from build123d import *

# Parameters (mm, degrees)
SKETCH_1_R      = 8.490267481
EXTRUDE_1_DEPTH = 2
SKETCH_2_R      = 1.25
EXTRUDE_2_DEPTH = 2.5


with BuildPart() as part:
    # Эскиз1 → Бобышка-Вытянуть1 (new body)
    with BuildSketch(Plane(origin=(0, 0, 0), x_dir=(1, 0, 0), z_dir=(0, 1, 0))):
        with Locations(Location((0, 0, 0), (0, 0, 270))):
            Circle(SKETCH_1_R)
        with BuildLine():
            Line((5.565646409, 0), (-5.565646409, 0))
            ThreePointArc((-5.565646409, 0), (-6.552289655, 0.474742908), (-6.796984316, 1.5419684))
            ThreePointArc((-6.796984316, 1.5419684), (0, 6.969696), (6.796984316, 1.5419684))
            ThreePointArc((6.796984316, 1.5419684), (6.552289655, 0.474742908), (5.565646409, 0))
        make_face(mode=Mode.SUBTRACT)
    extrude(amount=EXTRUDE_1_DEPTH)

    # Эскиз2 → Бобышка-Вытянуть2 (add)
    with BuildSketch(Plane.XZ):
        with Locations(Location((-4, 4.24513374, 0), (0, 0, 90))):
            Circle(SKETCH_2_R)
        with Locations(Location((4, 4.24513374, 0), (0, 0, 90))):
            Circle(SKETCH_2_R)
    extrude(amount=EXTRUDE_2_DEPTH)


solid = part.part
For this review, take the finished solid that the model builds, in its own axes (mm). A direction names the side the tool comes from. Coordinates: 2 decimals unless noted, no trailing zeros. Loops run counter-clockwise (first coordinate to the right, second up) from the corner with the lowest first, then second, coordinate; pieces in that order, holes last. Notation, with made-up numbers: (52, 7) - (89, 7) arc R21 cw to (89, 25) - close; hole circle Ø7 at (34.25, 8.5). An arc over 180 degrees is marked (long way). Use a Markdown table: item, result. Add a question column.
Item 1: We need section C-C (y = 1.5). Give the boundary of the cut face in (x, z), and give its area (3 significant figures).
Item 2: For line 1 (Z direction, x = 0.25, y = 1.35); line 2 (Y direction, x = -7, z = 4.5); line 3 (Z direction, x = 4, y = -0.65), list the stretches that pass through material, from the lowest coordinate up.
Item 3: We need section B-B (z = -2.5). Give the boundary of the cut face in (x, y).
Item 4: Tool access review of faces 4 (the face through (4.48, -1.23, 5.4)), 5 (the face through (0, 2, 2)), 6 (the face through (-6.54, 0.99, -0.46)): name each direction out of +Z, -Z, +X, -X, +Y, -Y from which nothing blocks a thin tool from reaching the whole face with its end or side.
Item 5: We need section A-A (x = 0). Give the boundary of the cut face in (y, z).
Item 6: We need section D-D (y = -1.1). Give the boundary of the cut face in (x, z).
Item 7: Insertion check: pin 1 Ø1.5 at (x, y) = (6.5, 0.5) entering from +Z; pin 2 Ø1.5 at (y, z) = (-0.5, -5) entering from -X; pin 3 Ø0.6 at (x, y) = (0.5, 1) entering from -Z. Each pin has a flat end and moves straight along its axis. Give the tip position at first contact, or say it passes through.
Item 8: Mouldability with a two-part tool opening along Z and no side actions: class faces 1 (the face through (-4, -2.5, 4)), 2 (the face through (0, 1, 0)), 3 (the face through (-3.52, -1.23, 5.4)) as pulls with the +Z half, pulls with the -Z half, needs draft (parallel to the pull), parting line crosses it, or undercut.
Results list:
| question | item | result |
|---|---|---|
| 1 | outline | circle Ø16.98 at (0, 0); hole (-6.8, -1.54) arc R6.97 ccw to (6.8, -1.54) arc R1.26 ccw to (5.57, 0) - (-5.57, 0) arc R1.26 ccw to start |
| 1 | area | 151 mm^2 |
| 2 | line 1 | z = -8.49 to -6.97, 0 to 8.49 |
| 2 | line 2 | y = 0 to 2 |
| 2 | line 3 | z = 3 to 5.5 |
| 3 | outline | (-8.11, 0) - (-6.51, 0) - (-6.51, 2) - (-8.11, 2) - close; (6.51, 0) - (8.11, 0) - (8.11, 2) - (6.51, 2) - close |
| 4 | face 4 | -Y |
| 4 | face 5 | +Z, -Z, +X, -X, +Y |
| 4 | face 6 | +Y, -Y |
| 5 | outline | (0, -8.49) - (2, -8.49) - (2, -6.97) - (0, -6.97) - close; (0, 0) - (2, 0) - (2, 8.49) - (0, 8.49) - close |
| 6 | outline | circle Ø2.5 at (-4, 4.25); circle Ø2.5 at (4, 4.25) |
| 7 | pin 1 | stops at z = 6.25 |
| 7 | pin 2 | stops at x = -7.24 |
| 7 | pin 3 | stops at z = -8.49 |
| 8 | face 1 | needs draft |
| 8 | face 2 | undercut |
| 8 | face 3 | parting line crosses it |
